CAD build for the part. Positions are in the model's coordinates, mm. A direction names the side the tool comes from. Give positions to 0.01 mm unless a question says otherwise; leave off trailing zeros. Loops run counter-clockwise (first coordinate to the right, second up) from the corner with the lowest first, then second, coordinate; pieces in that order, holes last. Notation, with made-up numbers: (27.25, 72) -> (63.25, 72) arc R14 cw to (63.25, 99) -> close; hole circle Ø2 at (-0.5, -16). An arc over 180 degrees is marked (long way). Use one line per item in the form item = value.
```python
from build123d import *

# Parameters (mm, degrees)
BOSS_EXTRUDE4_DEPTH = 50
FILLET1_R           = 10


with BuildPart() as part:
    # Sketch6 → Boss-Extrude4 (new body)
    with BuildSketch(Plane.XY):
        with BuildLine():
            Line((10, 0), (10, -20))
            ThreePointArc((10, -20), (10.585786438, -21.414213562), (12, -22))
            Line((12, -22), (37, -22))
            Line((37, -22), (37, -17))
            Line((37, -17), (17, -17))
            ThreePointArc((17, -17), (15.585786438, -16.414213562), (15, -15))
            Line((15, -15), (15, 0))
            ThreePointArc((15, 0), (0, 15), (-15, 0))
            Line((-15, 0), (-15, -15))
            ThreePointArc((-15, -15), (-15.585786438, -16.414213562), (-17, -17))
            Line((-17, -17), (-37, -17))
            Line((-37, -17), (-37, -22))
            Line((-37, -22), (-12, -22))
            ThreePointArc((-12, -22), (-10.585786438, -21.414213562), (-10, -20))
            Line((-10, -20), (-10, 0))
            ThreePointArc((-10, 0), (0, 10), (10, 0))
        make_face()
    extrude(amount=-BOSS_EXTRUDE4_DEPTH)

    # Fillet1
    fillet1_edges = [part.edges().sort_by_distance(p)[0] for p in [
        (37, -19.5, 0),
        (-37, -19.5, 0),
        (-37, -19.5, -50),
        (37, -19.5, -50),
    ]]
    fillet(fillet1_edges, radius=FILLET1_R)


solid = part.part
```
1. Cut at D-D, the plane x = 0. Write the cut outline in (y, z), then the cut area to 3 significant figures.
Result sheet:
outline = (10, -50) -> (15, -50) -> (15, 0) -> (10, 0) -> close
area = 250 mm^2
2. Mould opens along X. For faces 1 (the cylindrical face through (0, 10, -25)), 2 (the flat face through (37, -20, -25)), 3 (the flat face through (-27, -17, -25)) say: pulls with the +X half, pulls with the -X half, needs draft (parallel to the pull), parting line crosses it, or undercut.
Result sheet:
face_1 = undercut
face_2 = pulls with the +X half
face_3 = needs draft
3. Drop flat-ended pins along their axis: P1, Ø4, axis at x = 17.5, z = -34, coming from the +Y side; P2, Ø3, axis at y = -14.5, z = -18, coming from the +X side; P3, Ø6, axis at x = -28.5, z = -29.5, coming from the +Y side. Give the stop position or say it passes through.
Result sheet:
P1 = -16.32
P2 = 15.27
P3 = -17
4. Drill centre lines: line 1 (X direction, y = -9, z = -17); line 2 (Y direction, x = 18, z = -21); line 3 (X direction, y = -19, z = -29). Where is each one in solid material? Low to high.
Result sheet:
line_1 = -15 to -10, 10 to 15
line_2 = -22 to -17
line_3 = -37 to -10, 10 to 37
5. Cut at C-C, the plane y = -18. Write the cut outline in (x, z), then the cut area to 3 significant figures.
Result sheet:
outline = (-37, -40) arc R10 ccw to (-27, -50) -> (-10, -50) -> (-10, 0) -> (-27, 0) arc R10 ccw to (-37, -10) -> close; (10, -50) -> (27, -50) arc R10 ccw to (37, -40) -> (37, -10) arc R10 ccw to (27, 0) -> (10, 0) -> close
area = 2,610 mm^2
6. Cut at B-B, the plane z = -23. Write the cut outline in (x, y), then the cut area to 3 significant figures.
Result sheet:
outline = (-37, -22) -> (-12, -22) arc R2 ccw to (-10, -20) -> (-10, 0) arc R10 cw to (10, 0) -> (10, -20) arc R2 ccw to (12, -22) -> (37, -22) -> (37, -17) -> (17, -17) arc R2 cw to (15, -15) -> (15, 0) arc R15 ccw to (-15, 0) -> (-15, -15) arc R2 cw to (-17, -17) -> (-37, -17) -> close
area = 636 mm^2
7. Cut at A-A, the plane y = -9. Write the cut outline in (x, z), then the cut area to 3 significant figures.
Result sheet:
outline = (-15, -50) -> (-10, -50) -> (-10, 0) -> (-15, 0) -> close; (10, -50) -> (15, -50) -> (15, 0) -> (10, 0) -> close
area = 500 mm^2
8. Tool access for faces 4 (the flat face through (-15, -7, -25)), 5 (the flat face through (27, -17, -25)), 6 (the flat face through (-12, -5, -50)), 7 (the flat face through (-10, -10, -25)), 8 (the cylindrical face through (0, 15, -25)): list every direction of +Z, -Z, +X, -X, +Y, -Y with a clear straight run to the whole face (end or side of a thin tool).
Result sheet:
face_4 = +Z, -Z, -X, +Y
face_5 = +Z, -Z, +X, +Y
face_6 = -Z, +X, -X, +Y, -Y
face_7 = +Z, -Z, -Y
face_8 = +Z, -Z, +Y
